Drawing for the job (mm, zero at the part's lowest x, y, z). A direction names the side the tool comes from. Coordinates: 2 decimals unless noted, no trailing zeros. Write each loop counter-clockwise with the first axis right and the second up, starting at its lowest first coordinate (ties: lowest second). Pieces come first, ordered by that corner, then holes. Notation, with made-up numbers: M 55,10.25 L 99,10.25 A23 ccw 99,39.25 Z; hole C 4,-5.75 d9. An arc over 180 degrees is marked long. Use a Markdown table: item, result. Add a question column.
Q1. Slice it at D-D on x = 82.55. Write the cut outline in (y, z).
Q2. Slice it at A-A on x = 31.75. Write the cut outline in (y, z).
Q3. Mould opens along X. For the marked faces 1 and 2 say: released by +X, released by -X, zero draft, split by the parting line, or undercut.
Q4. Slice it at C-C on y = 3.5. Write the cut outline in (x, z) (1 decimal).
Q5. Tool access for the marked faces 3, 4, 5 and 6: list every direction of +Z, -Z, +X, -X, +Y, -Y with a clear straight run to the whole face (end or side of a thin tool).
Q6. Slice it at B-B on z = 12.7. Write the cut outline in (x, y).
Q7. Pin check, flat tips, straight feed: pin 1 Ø2.5 at (x, y) = (36.5, 8) entering from -Z; pin 2 Ø12 at (x, z) = (10.5, 14.5) entering from +Y; pin 3 Ø2 at (x, z) = (66, 8.5) entering from +Y; pin 4 Ø2 at (x, z) = (31.75, 12.7) entering from -Y. Stop position of each tip, or through.
Q8. Wall check: L1, parallel to X at y = 0.5, z = 12.7; L2, parallel to Y at x = 74, z = 14.75; L3, parallel to Z at x = 82.55, y = 0.55. Give the ranges that are in metal, low to high. Write a range as from..to.
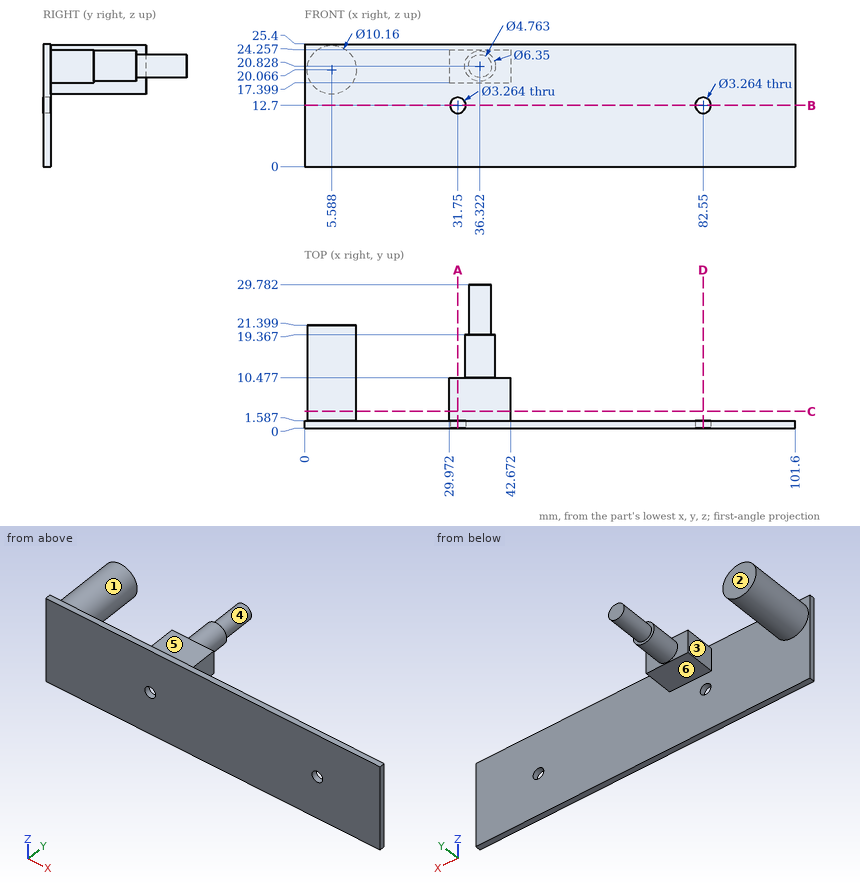
Recorded:
| question | item | result |
|---|---|---|
| 1 | outline | M 0,0 L 1.59,0 L 1.59,11.07 L 0,11.07 Z; M 0,14.33 L 1.59,14.33 L 1.59,25.4 L 0,25.4 Z |
| 2 | outline | M 0,0 L 1.59,0 L 1.59,11.07 L 0,11.07 Z; M 0,14.33 L 1.59,14.33 L 1.59,17.4 L 10.48,17.4 L 10.48,24.26 L 1.59,24.26 L 1.59,25.4 L 0,25.4 Z |
| 3 | face 1 | undercut |
| 3 | face 2 | zero draft |
| 4 | outline | C 5.6,20.1 d10.2; M 30,17.4 L 42.7,17.4 L 42.7,24.3 L 30,24.3 Z |
| 5 | face 3 | +Z, -Z, +Y |
| 5 | face 4 | +Y |
| 5 | face 5 | +Z, +X, +Y |
| 5 | face 6 | -Z, +X, +Y |
| 6 | outline | M 0,0 L 30.12,0 L 30.12,1.59 L 0,1.59 Z; M 33.38,0 L 80.92,0 L 80.92,1.59 L 33.38,1.59 Z; M 84.18,0 L 101.6,0 L 101.6,1.59 L 84.18,1.59 Z |
| 7 | pin 1 | z = 17.4 |
| 7 | pin 2 | y = 21.4 |
| 7 | pin 3 | y = 1.59 |
| 7 | pin 4 | through |
| 8 | L1 | 0..30.12, 33.38..80.92, 84.18..101.6 |
| 8 | L2 | 0..1.59 |
| 8 | L3 | 0..11.07, 14.33..25.4 |
